Verification items for the finished model (mm, model axes). Coordinates: 2 decimals unless noted, no trailing zeros. Loops run counter-clockwise (first coordinate to the right, second up) from the corner with the lowest first, then second, coordinate; pieces in that order, holes last. Notation, with made-up numbers: (48.25, 12.5) -> (81.25, 12.5) arc R24 ccw to (81.25, 44.5) -> close; hole circle Ø2 at (58.25, 68.5). An arc over 180 degrees is marked (long way). Write item = value, one per line.
```python
from build123d import *

# Parameters (mm, degrees)
F0_W     = 127
F0_H     = 101.6
F0_R     = 5.7277
F1_DEPTH = 25.4


with BuildPart() as f1:
    # F0 (on Front) → F1 (new body)
    with BuildSketch(Plane.XZ):
        Rectangle(F0_W, F0_H)
        with BuildLine():
            ThreePointArc((-38.1, 19.6723), (-42.150096, 29.450096), (-32.3723, 25.4))
            Line((-32.3723, 25.4), (-18.4277, 25.4))
            ThreePointArc((-18.4277, 25.4), (-12.7, 31.1277), (-6.9723, 25.4))
            Line((-6.9723, 25.4), (6.9723, 25.4))
            ThreePointArc((6.9723, 25.4), (12.7, 31.1277), (18.4277, 25.4))
            Line((18.4277, 25.4), (32.3723, 25.4))
            ThreePointArc((32.3723, 25.4), (38.1, 31.1277), (43.8277, 25.4))
            ThreePointArc((43.8277, 25.4), (42.150096, 21.349904), (38.1, 19.6723))
            Line((38.1, 19.6723), (38.1, 5.7277))
            ThreePointArc((38.1, 5.7277), (42.150096, 4.050096), (43.8277, 0))
            ThreePointArc((43.8277, 0), (42.150096, -4.050096), (38.1, -5.7277))
            Line((38.1, -5.7277), (38.1, -19.6723))
            ThreePointArc((38.1, -19.6723), (42.150096, -21.349904), (43.8277, -25.4))
            ThreePointArc((43.8277, -25.4), (38.1, -31.1277), (32.3723, -25.4))
            Line((32.3723, -25.4), (18.4277, -25.4))
            ThreePointArc((18.4277, -25.4), (12.7, -31.1277), (6.9723, -25.4))
            Line((6.9723, -25.4), (-6.9723, -25.4))
            ThreePointArc((-6.9723, -25.4), (-12.7, -31.1277), (-18.4277, -25.4))
            Line((-18.4277, -25.4), (-32.3723, -25.4))
            ThreePointArc((-32.3723, -25.4), (-42.150096, -29.450096), (-38.1, -19.6723))
            Line((-38.1, -19.6723), (-38.1, -5.7277))
            ThreePointArc((-38.1, -5.7277), (-43.8277, 0), (-38.1, 5.7277))
            Line((-38.1, 5.7277), (-38.1, 19.6723))
        make_face(mode=Mode.SUBTRACT)
        with BuildLine():
            Line((-18.4277, 25.4), (-32.3723, 25.4))
            ThreePointArc((-32.3723, 25.4), (-34.049904, 21.349904), (-38.1, 19.6723))
            Line((-38.1, 19.6723), (-38.1, 5.7277))
            ThreePointArc((-38.1, 5.7277), (-34.049904, 4.050096), (-32.3723, 0))
            ThreePointArc((-32.3723, 0), (-34.049904, -4.050096), (-38.1, -5.7277))
            Line((-38.1, -5.7277), (-38.1, -19.6723))
            ThreePointArc((-38.1, -19.6723), (-34.049904, -21.349904), (-32.3723, -25.4))
            Line((-32.3723, -25.4), (-18.4277, -25.4))
            ThreePointArc((-18.4277, -25.4), (-12.7, -19.6723), (-6.9723, -25.4))
            Line((-6.9723, -25.4), (6.9723, -25.4))
            ThreePointArc((6.9723, -25.4), (12.7, -19.6723), (18.4277, -25.4))
            Line((18.4277, -25.4), (32.3723, -25.4))
            ThreePointArc((32.3723, -25.4), (34.049904, -21.349904), (38.1, -19.6723))
            Line((38.1, -19.6723), (38.1, -5.7277))
            ThreePointArc((38.1, -5.7277), (32.3723, 0), (38.1, 5.7277))
            Line((38.1, 5.7277), (38.1, 19.6723))
            ThreePointArc((38.1, 19.6723), (34.049904, 21.349904), (32.3723, 25.4))
            Line((32.3723, 25.4), (18.4277, 25.4))
            ThreePointArc((18.4277, 25.4), (12.7, 19.6723), (6.9723, 25.4))
            Line((6.9723, 25.4), (-6.9723, 25.4))
            ThreePointArc((-6.9723, 25.4), (-12.7, 19.6723), (-18.4277, 25.4))
        make_face()
        with Locations((-12.7, 0)):
            Circle(F0_R, mode=Mode.SUBTRACT)
        with Locations((12.7, 0)):
            Circle(F0_R, mode=Mode.SUBTRACT)
    extrude(amount=F1_DEPTH)


solid = f1.part
```
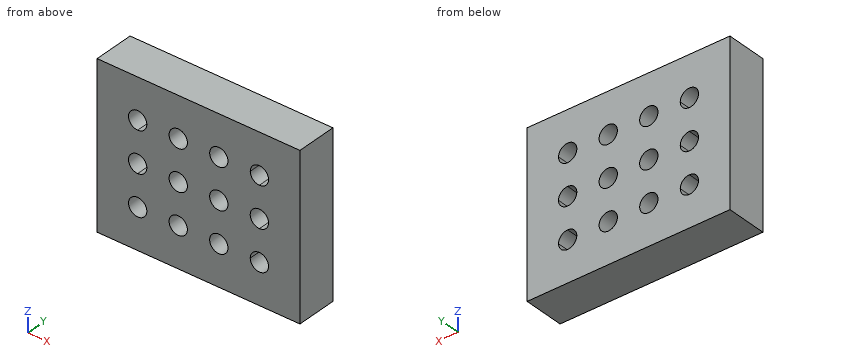
1) Sectioned sample at B-B, the plane x = -12.7. Record the cut outline in (y, z), plus the area to 3 significant figures.
Ans:
outline = (-25.4, -50.8) -> (0, -50.8) -> (0, -31.13) -> (-25.4, -31.13) -> close; (-25.4, -19.67) -> (0, -19.67) -> (0, -5.73) -> (-25.4, -5.73) -> close; (-25.4, 5.73) -> (0, 5.73) -> (0, 19.67) -> (-25.4, 19.67) -> close; (-25.4, 31.13) -> (0, 31.13) -> (0, 50.8) -> (-25.4, 50.8) -> close
area = 1,710 mm2
2) Material ranges on line 1 (X direction, y = -19.75, z = 25.4); line 2 (Z direction, x = -12.7, y = -17); line 3 (X direction, y = -21.75, z = -22.5), recorded low to high.
Ans:
line_1 = -63.5 to -43.83, -32.37 to -18.43, -6.97 to 6.97, 18.43 to 32.37, 43.83 to 63.5
line_2 = -50.8 to -31.13, -19.67 to -5.73, 5.73 to 19.67, 31.13 to 50.8
line_3 = -63.5 to -43.04, -33.16 to -17.64, -7.76 to 7.76, 17.64 to 33.16, 43.04 to 63.5
3) Depth check by flat-ended pin: pin 1 Ø3 at (x, z) = (10.5, -28) entering from +Y. Enter the tip coordinate at first touch or a pass-through.
Ans:
pin_1 = through
4) Sectioned sample at A-A, the plane y = -8.75. Count the separate pieces of the cut face and the enclosed holes in it, plus the area to 3 significant figures.
Ans:
separate_pieces = 1
enclosed_holes = 12
area = 11,700 mm2
